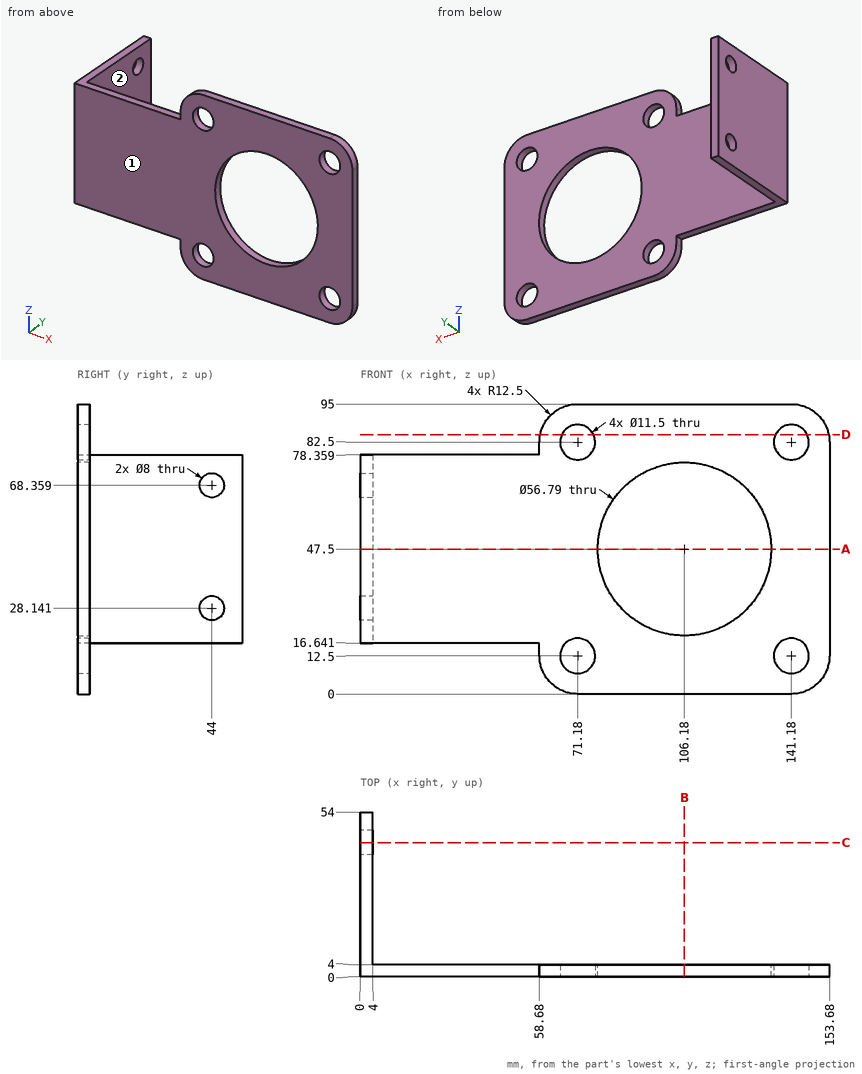
Study the drawing (mm; zero at the part's minimum x, y, z) and answer. A direction names the side the tool comes from. Round coordinates to 2 decimals unless told otherwise and drop trailing zeros. Order: outer loops, then holes, each group sorted by start corner. A loop starts at its lowest first (then second) coordinate and runs counter-clockwise, first axis right, second up. Notation, with made-up numbers: M 54,7 L 82,7 A33 cw 82,37 Z; hole C 9,63 d2. An arc over 180 degrees is marked long. One line per item, written item: value.
Q1. Find section D-D on z = 85. Write down the section's boundary in (x, y), then the cut area to 3 significant figures.
Derived:
outline: M 58.93,0 L 66,0 L 66,4 L 58.93,4 Z; M 76.36,0 L 136,0 L 136,4 L 76.36,4 Z; M 146.36,0 L 153.43,0 L 153.43,4 L 146.36,4 Z
area: 295 mm²
Q2. Find section B-B on x = 106.18. Write down the section's boundary in (y, z) (1 decimal), then the cut area to 3 significant figures.
Derived:
outline: M 0,0 L 4,0 L 4,19.1 L 0,19.1 Z; M 0,75.9 L 4,75.9 L 4,95 L 0,95 Z
area: 153 mm²
Q3. Flat-ended cylindrical pins translate along their axes: pin 1 (5 mm diameter, centred on x = 35, z = 38, fed in from +Y); pin 2 (25 mm diameter, centred on y = 36.5, z = 40, fed in from +X); pin 3 (3 mm diameter, centred on y = 1.5, z = 14, fed in from -X); pin 4 (7 mm diameter, centred on x = 141.18, z = 82.5, fed in from -Y). Find the tip coordinate at first contact, or state that the pin passes through.
Derived:
pin 1: y = 4
pin 2: x = 4
pin 3: x = 58.68
pin 4: through
Q4. Find section A-A on z = 47.5. Write down the section's boundary in (x, y) (1 decimal).
Derived:
outline: M 0,0 L 77.8,0 L 77.8,4 L 4,4 L 4,54 L 0,54 Z; M 134.6,0 L 153.7,0 L 153.7,4 L 134.6,4 Z
Q5. Straight lines are drawn through the part: line 1 (X direction, y = 1.7, z = 82.5); line 2 (Z direction, x = 141, y = 1); line 3 (Y direction, x = 98.5, z = 13). For each, find the intervals that lie inside material, in ascending order.
Derived:
line 1: 58.68 to 65.43, 76.93 to 135.43, 146.93 to 153.68
line 2: 0 to 6.75, 18.25 to 76.75, 88.25 to 95
line 3: 0 to 4
Q6. Find section C-C on y = 44. Write down the section's boundary in (x, z), then the cut area to 3 significant figures.
Derived:
outline: M 0,16.64 L 4,16.64 L 4,24.14 L 0,24.14 Z; M 0,32.14 L 4,32.14 L 4,64.36 L 0,64.36 Z; M 0,72.36 L 4,72.36 L 4,78.36 L 0,78.36 Z
area: 183 mm²
Q7. For the marked faces 1 and 2, determine the directions among +Z, -Z, +X, -X, +Y, -Y from which every point of the face is accessible in a straight line to the end or side of a thin tool.
Derived:
face 1: +Z, -Z, +X, -X, -Y
face 2: +Z, -Z, +X, +Y
